Part model, mm, in its own coordinate system. Give positions to 0.01 mm unless a question says otherwise; leave off trailing zeros. Write each loop counter-clockwise with the first axis right and the second up, starting at its lowest first coordinate (ties: lowest second). Pieces come first, ordered by that corner, then holes.
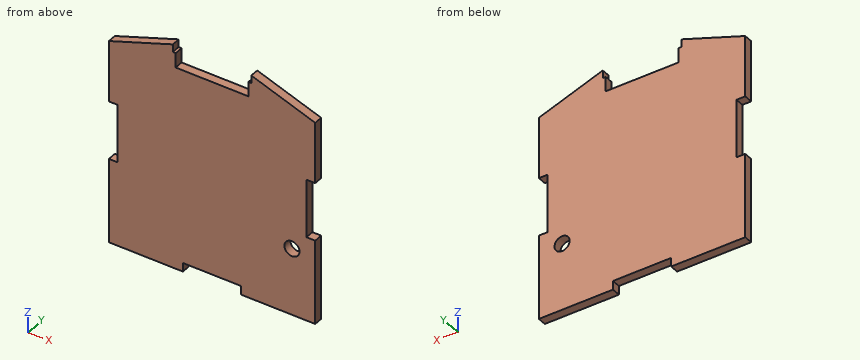
from build123d import *

# Parameters (mm, degrees)
F1_DEPTH = 3
F2_R     = 2.6
F3_DEPTH = 25


with BuildPart() as f1:
    # F0 (on Front) → F1 (new body)
    with BuildSketch(Plane.XZ):
        Polygon((-12.5, 31), (-35.5, 31), (-35.5, 10), (-32.5, 10), (-32.5, -10), (-35.5, -10), (-35.5, -39), (-10, -39), (-10, -36), (10, -36), (10, -39), (35.5, -39), (35.5, -10), (32.5, -10), (32.5, 10), (35.5, 10), (35.5, 31), (12.5, 31), align=None)
        Polygon((-13.5, 38.652174), (-35.5, 31), (-12.5, 31), (-12.5, 36), (-13.5, 36), align=None)
        Polygon((12.5, 36), (12.5, 31), (35.5, 31), (13.5, 38.652174), (13.5, 36), align=None)
    extrude(amount=F1_DEPTH)

    # F2 (on face) → F3 (cut)
    with BuildSketch(Plane.XZ.offset(3)):
        with Locations((27.5, -16)):
            Circle(F2_R)
    extrude(amount=-F3_DEPTH, mode=Mode.SUBTRACT)


solid = f1.part
1) Flat gauge pins, fed straight in: P1, Ø0.9, axis at x = -2.5, y = -1, coming from the -Z side; P2, Ø1.5, axis at x = 4, y = -2, coming from the +Z side; P3, Ø0.8, axis at x = -13, y = -1.5, coming from the +Z side. Where does each tip first touch, or does it go through?
Check result:
P1: stops at z = -36
P2: stops at z = 31
P3: stops at z = 36
2) Saw through at D-D (x = 17). Write the cut outline in (y, z).
Check result:
outline: (-3, -39) - (0, -39) - (0, 37.43) - (-3, 37.43) - close
3) Saw through at B-B (x = 28). Write the cut outline in (y, z).
Check result:
outline: (-3, -39) - (0, -39) - (0, -18.55) - (-3, -18.55) - close; (-3, -13.45) - (0, -13.45) - (0, 33.61) - (-3, 33.61) - close
4) Saw through at C-C (y = -0.8). Write the cut outline in (x, z).
Check result:
outline: (-35.5, -39) - (-10, -39) - (-10, -36) - (10, -36) - (10, -39) - (35.5, -39) - (35.5, -10) - (32.5, -10) - (32.5, 10) - (35.5, 10) - (35.5, 31) - (13.5, 38.65) - (13.5, 36) - (12.5, 36) - (12.5, 31) - (-12.5, 31) - (-12.5, 36) - (-13.5, 36) - (-13.5, 38.65) - (-35.5, 31) - (-35.5, 10) - (-32.5, 10) - (-32.5, -10) - (-35.5, -10) - close; hole circle Ø5.2 at (27.5, -16)
5) Saw through at A-A (z = -16). Write the cut outline in (x, y), and give its area (3 significant figures).
Check result:
outline: (-35.5, -3) - (24.9, -3) - (24.9, 0) - (-35.5, 0) - close; (30.1, -3) - (35.5, -3) - (35.5, 0) - (30.1, 0) - close
area: 197 mm2
6) Drill centre lines: L1, parallel to Z at x = 27.5, y = -1; L2, parallel to Z at x = -5, y = -0.8; L3, parallel to X at y = -2.25, z = 6. Where is each one in solid material? Low to high.
Check result:
L1: z = -39 to -18.6, -13.4 to 33.78
L2: z = -36 to 31
L3: x = -32.5 to 32.5
